Model file for the job. Use its own axes, mm. Face numbers are marked on the shaded views. Give positions to 0.01 mm unless a question says otherwise; leave off trailing zeros. Write each loop counter-clockwise with the first axis right and the second up, starting at its lowest first coordinate (ties: lowest second). Pieces come first, ordered by that corner, then holes.
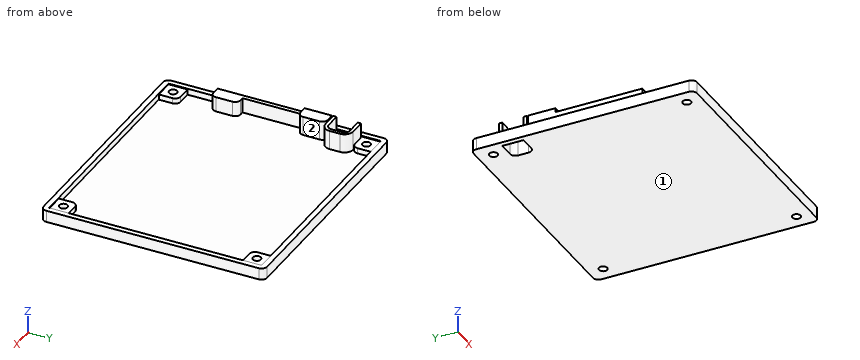
```python
from build123d import *

# Parameters (mm, degrees)
F1_DEPTH  = 2
F2_W      = 86
F2_H      = 78
F3_DEPTH  = 2.3
F5_DEPTH  = 2
F6_R      = 1.5
F7_DEPTH  = 6
F9_DEPTH  = 7
F11_DEPTH = 5.5
F13_DEPTH = 25
F15_DEPTH = 7
F16_W     = 1.6
F16_H     = 22
F17_DEPTH = 5.5


with BuildPart() as f1:
    # F0 (on Top) → F1 (new body)
    with BuildSketch(Plane.XY):
        with BuildLine():
            ThreePointArc((0, 2), (0.585786, 0.585786), (2, 0))
            Line((2, 0), (88, 0))
            ThreePointArc((88, 0), (89.414214, 0.585786), (90, 2))
            Line((90, 2), (90, 80))
            ThreePointArc((90, 80), (89.414214, 81.414214), (88, 82))
            Line((88, 82), (2, 82))
            ThreePointArc((2, 82), (0.585786, 81.414214), (0, 80))
            Line((0, 80), (0, 2))
        make_face()
    extrude(amount=F1_DEPTH)

    # F2 (on face) → F3 (join)
    with BuildSketch(Plane.XY.offset(2)):
        with BuildLine():
            ThreePointArc((2, 82), (0.585786, 81.414214), (0, 80))
            Line((0, 80), (0, 2))
            ThreePointArc((0, 2), (0.585786, 0.585786), (2, 0))
            Line((2, 0), (88, 0))
            ThreePointArc((88, 0), (89.414214, 0.585786), (90, 2))
            Line((90, 2), (90, 80))
            ThreePointArc((90, 80), (89.414214, 81.414214), (88, 82))
            Line((88, 82), (2, 82))
        make_face()
        with Locations((45, 41)):
            Rectangle(F2_W, F2_H, mode=Mode.SUBTRACT)
    extrude(amount=F3_DEPTH)

    # F4 (on face) → F5 (join)
    with BuildSketch(Plane.XY.offset(2)):
        with BuildLine():
            Line((2, 9), (2, 2))
            Line((2, 2), (9, 2))
            Line((9, 2), (9, 7))
            ThreePointArc((9, 7), (8.414214, 8.414214), (7, 9))
            Line((7, 9), (2, 9))
        make_face()
        with BuildLine():
            Line((9, 80), (2, 80))
            Line((2, 80), (2, 73))
            Line((2, 73), (7, 73))
            ThreePointArc((7, 73), (8.414214, 73.585786), (9, 75))
            Line((9, 75), (9, 80))
        make_face()
        with BuildLine():
            Line((81, 2), (88, 2))
            Line((88, 2), (88, 9))
            Line((88, 9), (83, 9))
            ThreePointArc((83, 9), (81.585786, 8.414214), (81, 7))
            Line((81, 7), (81, 2))
        make_face()
        with BuildLine():
            Line((88, 73), (88, 80))
            Line((88, 80), (81, 80))
            Line((81, 80), (81, 75))
            ThreePointArc((81, 75), (81.585786, 73.585786), (83, 73))
            Line((83, 73), (88, 73))
        make_face()
    extrude(amount=F5_DEPTH)

    # F6 (on face) → F7 (cut)
    with BuildSketch(Plane(origin=(0, 0, 0), x_dir=(1, 0, 0), z_dir=(0, 0, -1))):
        with Locations((84.5, -5.5)):
            Circle(F6_R)
        with Locations((84.5, -76.5)):
            Circle(F6_R)
        with Locations((5.5, -76.5)):
            Circle(F6_R)
        with Locations((5.5, -5.5)):
            Circle(F6_R)
    extrude(amount=-F7_DEPTH, mode=Mode.SUBTRACT)

    # F8 (on face) → F9 (join)
    with BuildSketch(Plane.XY.offset(2)):
        with BuildLine():
            Line((5, 62), (2, 62))
            Line((2, 62), (2, 52))
            Line((2, 52), (5, 52))
            ThreePointArc((5, 52), (6.414214, 52.585786), (7, 54))
            Line((7, 54), (7, 60))
            ThreePointArc((7, 60), (6.414214, 61.414214), (5, 62))
        make_face()
    extrude(amount=F9_DEPTH)

    # F10 (on face) → F11 (join)
    with BuildSketch(Plane.XY.offset(2)):
        with BuildLine():
            Line((2, 30), (2, 20))
            Line((2, 20), (5, 20))
            ThreePointArc((5, 20), (6.414214, 20.585786), (7, 22))
            Line((7, 22), (7, 28))
            ThreePointArc((7, 28), (6.414214, 29.414214), (5, 30))
            Line((5, 30), (2, 30))
        make_face()
    extrude(amount=F11_DEPTH)

    # F12 (on face) → F13 (cut)
    with BuildSketch(Plane(origin=(0, 0, 0), x_dir=(1, 0, 0), z_dir=(0, 0, -1))):
        with BuildLine():
            Line((2, -63.7), (2, -71.5))
            Line((2, -71.5), (7.6, -71.5))
            ThreePointArc((7.6, -71.5), (9.014214, -70.914214), (9.6, -69.5))
            Line((9.6, -69.5), (9.6, -65.7))
            ThreePointArc((9.6, -65.7), (9.014214, -64.285786), (7.6, -63.7))
            Line((7.6, -63.7), (2, -63.7))
        make_face()
    extrude(amount=-F13_DEPTH, mode=Mode.SUBTRACT)

    # F14 (on face) → F15 (join)
    with BuildSketch(Plane.XY.offset(2)):
        with BuildLine():
            ThreePointArc((10.8, 69.5), (9.862742, 71.762742), (7.6, 72.7))
            Line((7.6, 72.7), (2, 72.7))
            Line((2, 72.7), (2, 71.5))
            Line((2, 71.5), (7.6, 71.5))
            ThreePointArc((7.6, 71.5), (9.014214, 70.914214), (9.6, 69.5))
            Line((9.6, 69.5), (9.6, 65.7))
            ThreePointArc((9.6, 65.7), (9.014214, 64.285786), (7.6, 63.7))
            Line((7.6, 63.7), (2, 63.7))
            Line((2, 63.7), (2, 62.5))
            Line((2, 62.5), (7.6, 62.5))
            ThreePointArc((7.6, 62.5), (9.862742, 63.437258), (10.8, 65.7))
            Line((10.8, 65.7), (10.8, 69.5))
        make_face()
    extrude(amount=F15_DEPTH)

    # F16 (on face) → F17 (join)
    with BuildSketch(Plane.XY.offset(2)):
        with Locations((2.8, 41)):
            Rectangle(F16_W, F16_H)
    extrude(amount=F17_DEPTH)


solid = f1.part
```
1. Probe probe 1 along X at (y, z) = (5.5, 3.25); probe 2 along X at (y, z) = (5.5, 1.1); probe 3 along Y at (x, z) = (84.5, 2.4). List the from-to ranges inside material, lowest first.
Calculated:
probe 1: x = 0 to 4, 7 to 9, 81 to 83, 86 to 90
probe 2: x = 0 to 4, 7 to 83, 86 to 90
probe 3: y = 0 to 4, 7 to 9, 73 to 75, 78 to 82
2. Slice it at A-A, the plane y = 5.5. Write the cut outline in (x, z).
Calculated:
outline: (0, 0) - (4, 0) - (4, 4) - (2, 4) - (2, 4.3) - (0, 4.3) - close; (7, 0) - (83, 0) - (83, 4) - (81, 4) - (81, 2) - (9, 2) - (9, 4) - (7, 4) - close; (86, 0) - (90, 0) - (90, 4.3) - (88, 4.3) - (88, 4) - (86, 4) - close
3. Slice it at D-D, the plane y = 41. Write the cut outline in (x, z).
Calculated:
outline: (0, 0) - (90, 0) - (90, 4.3) - (88, 4.3) - (88, 2) - (3.6, 2) - (3.6, 7.5) - (2, 7.5) - (2, 4.3) - (0, 4.3) - close
4. Slice it at C-C, the plane z = 6. Write the cut outline in (x, y).
Calculated:
outline: (2, 20) - (5, 20) arc R2 ccw to (7, 22) - (7, 28) arc R2 ccw to (5, 30) - (3.6, 30) - (3.6, 52) - (5, 52) arc R2 ccw to (7, 54) - (7, 60) arc R2 ccw to (5, 62) - (2, 62) - close; (2, 62.5) - (7.6, 62.5) arc R3.2 ccw to (10.8, 65.7) - (10.8, 69.5) arc R3.2 ccw to (7.6, 72.7) - (2, 72.7) - (2, 71.5) - (7.6, 71.5) arc R2 cw to (9.6, 69.5) - (9.6, 65.7) arc R2 cw to (7.6, 63.7) - (2, 63.7) - close
5. Slice it at B-B, the plane x = 84.5. Write the cut outline in (y, z).
Calculated:
outline: (0, 0) - (4, 0) - (4, 4) - (2, 4) - (2, 4.3) - (0, 4.3) - close; (7, 0) - (75, 0) - (75, 4) - (73, 4) - (73, 2) - (9, 2) - (9, 4) - (7, 4) - close; (78, 0) - (82, 0) - (82, 4.3) - (80, 4.3) - (80, 4) - (78, 4) - close
6. Pull direction Y, two halves, no side cores. Call the marked faces 1 and 2: +Y half, -Y half, draft (parallel to the pull), parting line (faces both ways), or undercut.
Calculated:
face 1: draft
face 2: undercut
7. Pin check, flat tips, straight feed: P1, Ø3.5, axis at x = 85.5, y = 4, coming from the +Z side; P2, Ø4, axis at y = 14.5, z = 8, coming from the -X side; P3, Ø12, axis at x = 22.5, y = 41.5, coming from the +Z side; P4, Ø2.5, axis at y = 48, z = 7, coming from the -X side. Stop position of each tip, or through.
Calculated:
P1: stops at z = 4
P2: passes through
P3: stops at z = 2
P4: stops at x = 2
